Read the model definition and answer for the solid it produces. Units are mm, in the model's axes. A direction names the side the tool comes from. Round coordinates to 2 decimals unless told otherwise and drop trailing zeros. Order: outer loops, then holes, each group sorted by start corner. A loop starts at its lowest first (then second) coordinate and runs counter-clockwise, first axis right, second up.
from build123d import *

# Parameters (mm, degrees)
F0_W     = 15.875
F0_H     = 3.175
F1_DEPTH = 5.5626
F2_W     = 15.875
F2_H     = 2.54
F3_DEPTH = 4.7752
F4_W     = 1.016
F4_H     = 3.175
F5_DEPTH = 0.508
F6_W     = 0.9525
F6_H     = 3.175
F6_W_2   = 1.016
F7_DEPTH = 1.143


with BuildPart() as f1:
    # F0 (on Top) → F1 (new body)
    with BuildSketch(Plane.XY):
        Rectangle(F0_W, F0_H)
    extrude(amount=F1_DEPTH)

    # F2 (on face) → F3 (join)
    with BuildSketch(Plane(origin=(0, 1.5875, 0), x_dir=(-1, 0, 0), z_dir=(0, 1, 0))):
        with Locations((0, 4.2926)):
            Rectangle(F2_W, F2_H)
    extrude(amount=F3_DEPTH)

    # F4 (on face) → F5 (join)
    with BuildSketch(Plane(origin=(0, 0, 0), x_dir=(1, 0, 0), z_dir=(0, 0, -1))):
        Rectangle(F4_W, F4_H)
    extrude(amount=F5_DEPTH)

    # F6 (on face) → F7 (join)
    with BuildSketch(Plane(origin=(0, 0, -0.508), x_dir=(1, 0, 0), z_dir=(0, 0, -1))):
        with Locations((0.98425, 0)):
            Rectangle(F6_W, F6_H)
        Rectangle(F6_W_2, F6_H)
        with Locations((-0.98425, 0)):
            Rectangle(F6_W, F6_H)
    extrude(amount=F7_DEPTH)


solid = f1.part
Q1. For faces 1 (the face through (1.46, 0, -1)), 2 (the face through (-1.46, 0, -1)), 3 (the face through (-1, 0, -0.508)), determine the directions among +Z, -Z, +X, -X, +Y, -Y from which every point of the face is accessible in a straight line to the end or side of a thin tool.
Outcome:
face 1: -Z, +X, +Y, -Y
face 2: -Z, -X, +Y, -Y
face 3: -X, +Y, -Y
Q2. For a pull along Z with two mould halves and no side action, classify faces 4 (the face through (1, 0, -0.508)), 5 (the face through (0, -1.588, 3)), 6 (the face through (0, 0, -1.651)) as released by +Z, released by -Z, zero draft, split by the parting line, or undercut.
Outcome:
face 4: undercut
face 5: zero draft
face 6: released by -Z
Q3. A cutting plane is placed at D-D, the plane z = 0.75. Give the vertices of the cut face in (x, y).
Outcome:
outline: (-7.94, -1.59) - (7.94, -1.59) - (7.94, 1.59) - (-7.94, 1.59) - close
Q4. A cutting plane is placed at B-B, the plane y = 0.5. Give the vertices of the cut face in (x, z), plus the area to 3 significant figures.
Outcome:
outline: (-7.94, 0) - (-0.51, 0) - (-0.51, -0.51) - (-1.46, -0.51) - (-1.46, -1.65) - (1.46, -1.65) - (1.46, -0.51) - (0.51, -0.51) - (0.51, 0) - (7.94, 0) - (7.94, 5.56) - (-7.94, 5.56) - close
area: 92.2 mm2
Q5. Flat-ended cylindrical pins translate along their axes: pin 1 (1 mm diameter, centred on x = 5, y = 2, fed in from -Z); pin 2 (1.3 mm diameter, centred on y = 0, z = -1, fed in from -X); pin 3 (3.5 mm diameter, centred on x = -3.5, z = 0.5, fed in from +Y). Find the tip coordinate at first contact, or state that the pin passes through.
Outcome:
pin 1: stops at z = 0
pin 2: stops at x = -1.46
pin 3: stops at y = 1.59
Q6. Straight lines are drawn through the part: probe 1 along Z at (x, y) = (-7, 2); probe 2 along Y at (x, z) = (1, 2); probe 3 along Z at (x, y) = (5.75, 0.25). For each, find the intervals that lie inside material, in ascending order.
Outcome:
probe 1: z = 3.02 to 5.56
probe 2: y = -1.59 to 1.59
probe 3: z = 0 to 5.56
Q7. A cutting plane is placed at A-A, the plane x = -1. Give the vertices of the cut face in (y, z), plus the area to 3 significant figures.
Outcome:
outline: (-1.59, -1.65) - (1.59, -1.65) - (1.59, -0.51) - (-1.59, -0.51) - close; (-1.59, 0) - (1.59, 0) - (1.59, 3.02) - (6.36, 3.02) - (6.36, 5.56) - (-1.59, 5.56) - close
area: 33.4 mm2
Q8. A cutting plane is placed at C-C, the plane x = -4.5. Give the vertices of the cut face in (y, z).
Outcome:
outline: (-1.59, 0) - (1.59, 0) - (1.59, 3.02) - (6.36, 3.02) - (6.36, 5.56) - (-1.59, 5.56) - close
